Could you check a few things on this model? Use its own coordinates, in mm. A direction names the side the tool comes from. Give positions to 0.01 mm unless a question says otherwise; leave off trailing zeros. Loops run counter-clockwise (first coordinate to the right, second up) from the corner with the lowest first, then second, coordinate; pieces in that order, holes last. Notation, with made-up numbers: M 72.5,-2.5 L 109.5,-2.5 A33 ccw 109.5,26.5 Z; hole C -8.75,-9.75 d11. An arc over 180 degrees is marked long. Use a Markdown table: item, result. Add a question column.
1) We'd pull the mould along Z, two halves only. Please class faces 1 (the flat face through (-0.49, 8.16, -0.87)), 2 (the cylindrical face through (-0.29, 7.38, 2.23)), 3 (the flat face through (1, 8.7, -1)): +Z half, -Z half, draft (parallel to the pull), parting line (faces both ways), or undercut.
2) Suppose I cut it at B-B on y = 3. List the corners of the cut face in (x, z) for me.
3) Suppose I cut it at A-A on y = 0.75. List the corners of the cut face in (x, z) for me, and give its area (3 significant figures).
4) Which directions (+Z, -Z, +X, -X, +Y, -Y) give clear straight access to the entire face, cutting with the end or side of a thin tool? Please do faces 4 (the flat face through (-1, 0, 1)), 5 (the flat face through (-2, 4, 0)), 6 (the flat face through (-0.51, 8.16, 0.86)).
5) Will these pins go through, and if not, where does the flat tip stop? pin 1 Ø1.5 at (x, y) = (-1.5, 3.5) entering from +Z; pin 2 Ø0.5 at (y, z) = (8.5, -0.5) entering from -X.
6) If I drill on line 1 along Y through (x, z) = (1.65, 1.25); line 2 along Y through (x, z) = (0.1, 1.7); line 3 along X through (y, z) = (7.75, 0.5), over which ranges is the centre line in solid material (lowest first)? Write a range as [from, to].
Autodesk Inventor part; units mm, degrees
ref_plane "AS_XY" through (0, 8.7, 0) normal (0, 1, 0) x (1, 0, 0)
ref_plane "AS_YZ" through (0, 8.7, 0) normal (1, 0, 0) x (0, 0, -1)
ref_plane "AS_ZX" through (0, 8.7, 0) normal (0, 0, -1) x (0, 1, 0)
sketch "Sketch_3" plane through (0, 0, 0) normal (1, 0, 0) x (0, 1, 0)
  line L0 (1, 0) -> (0, 0)
  line L1 (0, 0) -> (0, 2.2)
  line L2 (0, 2.2) -> (0.05, 2.25)
  line L3 (0.05, 2.25) -> (0.95, 2.25)
  line L4 (0.95, 2.25) -> (1, 2.2)
  line L5 (1, 2.2) -> (1, 0)
  line L6 (1, 0) -> (0, 0)
revolve "Revolution1" add sketch "Sketch_3" angle 360 about axis through (0, 1, 0) along (0, 1, 0)
sketch "Sketch_9" plane through (0, 0, 0) normal (1, 0, 0) x (0, 1, 0)
  line L0 (-100, 0) -> (100, 0)
  line L1 (6.3, -1.25) -> (1, -1.25)
  line L2 (1, -1.25) -> (1, -2.2)
  line L3 (1, -2.2) -> (1.05, -2.25)
  line L4 (1.05, -2.25) -> (1.7, -2.25)
  line L5 (1.7, -2.25) -> (1.7, -1.75)
  line L6 (1.7, -1.75) -> (4, -1.75)
  line L7 (4, -1.75) -> (4, -2.25)
  line L8 (4, -2.25) -> (6.25, -2.25)
  line L9 (6.25, -2.25) -> (6.3, -2.2)
  line L10 (6.3, -2.2) -> (6.3, -1.25)
revolve "Revolution2" add sketch "Sketch_9" angle 360 about axis through (0, -100, 0) along (0, -1, 0)
sketch "Sketch_6" plane through (0, 0, 0) normal (0, 0, 1) x (1, 0, 0)
  line L0 (0, -50) -> (0, 50)
  line L1 (0, 8.7) -> (2.05, 8.7)
  arc A0 (2.25, 8.5) -> (2.05, 8.7) centre (2.05, 8.5) ccw
  line L2 (2.25, 8.5) -> (2.25, 6.3)
  line L3 (2.25, 6.3) -> (0, 6.3)
  line L4 (0, 6.3) -> (0, 8.7)
revolve "Revolution3" add sketch "Sketch_6" angle 360 about axis through (0, -50, 0) along (0, -1, 0)
sketch "Sketch_7" plane through (0, 8.7, 0) normal (0, 1, 0) x (1, 0, 0)
  line L0 (-1, -0.5774) -> (0, -1.1547)
  line L1 (0, -1.1547) -> (1, -0.5774)
  line L2 (1, -0.5774) -> (1, 0.5774)
  line L3 (1, 0.5774) -> (0, 1.1547)
  line L4 (0, 1.1547) -> (-1, 0.5774)
  line L5 (-1, 0.5774) -> (-1, -0.5774)
extrude "Extrusion1" cut sketch "Sketch_7" against normal blind 1.1
sketch "Sketch_10" plane through (0, 0, 0) normal (1, 0, 0) x (0, 1, 0)
  line L0 (-3.7, 0) -> (6.3, 0)
  line L1 (6.3, 0) -> (6.3, -1.25)
  line L2 (6.3, -1.25) -> (-3.424, -1.25)
  line L3 (-3.424, -1.25) -> (-3.7, -0.974)
  line L4 (-3.7, -0.974) -> (-3.7, 0)
  line L5 (-3.7, 0) -> (6.3, 0)
revolve "Revolution4" add sketch "Sketch_10" angle 360 about axis through (0, -3.7, 0) along (0, -1, 0)
thread "Thread1"
ref_plane "AS_XY" through (0, 8.7, 0) normal (0, 1, 0) x (1, 0, 0)
ref_plane "AS_YZ" through (0, 8.7, 0) normal (1, 0, 0) x (0, 0, -1)
ref_plane "AS_ZX" through (0, 8.7, 0) normal (0, 0, -1) x (0, 1, 0)
ref_plane "hul_XY" through (0, 0, 0) normal (0, 1, 0) x (1, 0, 0)
ref_plane "hul_YZ" through (0, 0, 0) normal (1, 0, 0) x (0, 0, -1)
ref_plane "hul_ZX" through (0, 0, 0) normal (0, 0, -1) x (0, 1, 0)
ref_plane "s01_XY" through (0, 5.3, 0) normal (0, 1, 0) x (1, 0, 0)
ref_plane "s01_YZ" through (0, 5.3, 0) normal (1, 0, 0) x (0, 0, -1)
ref_plane "s01_ZX" through (0, 5.3, 0) normal (0, 0, -1) x (0, 1, 0)
properties part number "SCHUNK-5509536 Huelse MPG 40"
Answer block:
| question | item | result |
|---|---|---|
| 1 | face 1 | undercut |
| 1 | face 2 | parting line |
| 1 | face 3 | draft |
| 2 | outline | C 0,0 d3.5 |
| 3 | outline | C 0,0 d4.5 |
| 3 | area | 15.9 mm^2 |
| 4 | face 4 | -Y |
| 4 | face 5 | none |
| 4 | face 6 | +Y |
| 5 | pin 1 | stops at z = 2.04 |
| 5 | pin 2 | stops at x = -2.24 |
| 6 | line 1 | y = [0, 1.7], [4, 8.7] |
| 6 | line 2 | y = [0, 8.7] |
| 6 | line 3 | x = [-2.19, -1], [1, 2.19] |
